from build123d import *

# Parameters (mm, degrees)
SKETCH1_W            = 300
SKETCH1_H            = 200
BOSS_EXTRUDE1_DEPTH  = 6
SKETCH6_R            = 2.5
CUT_EXTRUDE2_DEPTH   = 7
FILLET1_R            = 6.35
SKETCH16_R           = 3.25
M5_TAP2_DEPTH        = 7
SKETCH17_R           = 1.25
SKETCH17_R_2         = 3.175
SKETCH17_R_3         = 4.7625
M3_COUNTERBORE_DEPTH = 7
CUT_EXTRUDE6_DEPTH   = 7
SKETCH19_R           = 1.25
CUT_EXTRUDE7_DEPTH   = 7


with BuildPart() as part:
    # Sketch1 → Boss-Extrude1 (new body)
    with BuildSketch(Plane(origin=(0, 0, 0), x_dir=(1, 0, 0), z_dir=(0, 1, 0))):
        with Locations((150, 100)):
            Rectangle(SKETCH1_W, SKETCH1_H)
    extrude(amount=BOSS_EXTRUDE1_DEPTH)

    # Sketch6 → Cut-Extrude2 (cut, through all)
    with BuildSketch(Plane(origin=(0, 6, 0), x_dir=(1, 0, 0), z_dir=(0, 1, 0))):
        with Locations((150, 118.65102)):
            Circle(SKETCH6_R)
    extrude(amount=-CUT_EXTRUDE2_DEPTH, mode=Mode.SUBTRACT)

    # Fillet1
    fillet1_edges = [part.edges().sort_by_distance(p)[0] for p in [
        (0, 3, -200),
        (300, 3, -200),
        (300, 3, 0),
        (0, 3, 0),
    ]]
    fillet(fillet1_edges, radius=FILLET1_R)

    # Sketch16 → M5-tap2 (cut, through all)
    with BuildSketch(Plane(origin=(0, 6, -5.8), x_dir=(1, 0, 0), z_dir=(0, -1, 0))):
        with Locations((118.25, -18.65102)):
            Circle(SKETCH16_R)
        with Locations((139.416666667, -0.55098)):
            Circle(SKETCH16_R)
        with Locations((160.583333333, -0.55098)):
            Circle(SKETCH16_R)
        with Locations((181.75, -18.65102)):
            Circle(SKETCH16_R)
    extrude(amount=M5_TAP2_DEPTH, mode=Mode.SUBTRACT)

    # Sketch17 → M3_counterbore (cut, through all)
    with BuildSketch(Plane(origin=(0, 6, 0), x_dir=(1, 0, 0), z_dir=(0, 1, 0))):
        with Locations((185, 118.65102)):
            Circle(SKETCH17_R)
        with Locations((167.5, 88.340130868)):
            Circle(SKETCH17_R)
        with Locations((132.5, 88.340130868)):
            Circle(SKETCH17_R)
        with Locations((115, 118.65102)):
            Circle(SKETCH17_R)
        with Locations((132.5, 148.961909132)):
            Circle(SKETCH17_R)
        with Locations((167.5, 148.961909132)):
            Circle(SKETCH17_R)
        with Locations((150, 138.65102)):
            Circle(SKETCH17_R_2)
        with Locations((167.320508076, 128.65102)):
            Circle(SKETCH17_R_2)
        with Locations((167.320508076, 108.65102)):
            Circle(SKETCH17_R_2)
        with Locations((150, 98.65102)):
            Circle(SKETCH17_R_2)
        with Locations((132.679491924, 108.65102)):
            Circle(SKETCH17_R_2)
        with Locations((132.679491924, 128.65102)):
            Circle(SKETCH17_R_2)
        with Locations((160, 135.971528076)):
            Circle(SKETCH17_R_3)
        with Locations((170, 118.65102)):
            Circle(SKETCH17_R_3)
        with Locations((160, 101.330511924)):
            Circle(SKETCH17_R_3)
        with Locations((140, 101.330511924)):
            Circle(SKETCH17_R_3)
        with Locations((130, 118.65102)):
            Circle(SKETCH17_R_3)
        with Locations((140, 135.971528076)):
            Circle(SKETCH17_R_3)
    extrude(amount=-M3_COUNTERBORE_DEPTH, mode=Mode.SUBTRACT)

    # Sketch18 → Cut-Extrude6 (cut, through all)
    with BuildSketch(Plane(origin=(0, 6, 0), x_dir=(1, 0, 0), z_dir=(0, 1, 0))):
        Polygon((154.8, 121.422301292), (154.8, 115.879738708), (150, 113.108457416), (145.2, 115.879738708), (145.2, 121.422301292), (150, 124.193582584), align=None)
    extrude(amount=-CUT_EXTRUDE6_DEPTH, mode=Mode.SUBTRACT)

    # Sketch19 → Cut-Extrude7 (cut, through all)
    with BuildSketch(Plane(origin=(0, 6, 0), x_dir=(1, 0, 0), z_dir=(0, 1, 0))):
        with Locations((118.25, 15.401)):
            Circle(SKETCH19_R)
        with Locations((150, 6.35098)):
            Circle(SKETCH19_R)
        with Locations((181.75, 15.401)):
            Circle(SKETCH19_R)
    extrude(amount=-CUT_EXTRUDE7_DEPTH, mode=Mode.SUBTRACT)


solid = part.part
Model file for the job. Use its own axes, mm. A direction names the side the tool comes from. Give positions to 0.01 mm unless a question says otherwise; leave off trailing zeros.
1) Tool access for faces 1 (the flat face through (147.9, 0, -101.4)), 2 (the flat face through (154.8, 3, -119)): list every direction of +Z, -Z, +X, -X, +Y, -Y with a clear straight run to the whole face (end or side of a thin tool).
2) Wall check: line 1 (X direction, y = 5.1, z = -109); line 2 (Z direction, x = 150, y = 3.2); line 3 (Z direction, x = 160, y = 3.4). Give the ranges that are in metal, low to high.
3) Saw through at A-A (y = 3.35). Count the separate pieces of the cut face and the enclosed holes in it, plus the area to 3 significant figures.
4) Flat gauge pin, fed straight in: pin 1 Ø4 at (x, z) = (160.58, -6.35) entering from -Y. Where does the tip first touch, or does it go through?
5) Pull direction Z, two halves, no side cores. Call faces 3 (the flat face through (148, 3, -200)), 4 (the flat face through (300, 3, -99)), 5 (the cylindrical face through (1.81, 3.04, -1.91)), 6 (the cylindrical face through (159.38, 3.042, -106.052)): +Z half, -Z half, draft (parallel to the pull), parting line (faces both ways), or undercut.
Answer block:
1. face 1: +Z, -Z, +X, -X, -Y
1. face 2: +Y, -Y
2. line 1: x = 0 to 129.52, 135.84 to 164.16, 170.48 to 300
2. line 2: z = -200 to -141.83, -135.48 to -124.19, -113.11 to -101.83, -95.48 to -7.6, -5.1 to 0
2. line 3: z = -200 to -140.73, -131.21 to -106.09, -96.57 to -9.55, -3.15 to 0
3. separate pieces: 1
3. enclosed holes: 26
3. area: 59,100 mm2
4. pin 1: passes through
5. face 3: -Z half
5. face 4: draft
5. face 5: +Z half
5. face 6: undercut
